Read the model definition and answer for the solid it produces. Units are mm, in the model's axes. Face numbers are marked on the shaded views. A direction names the side the tool comes from. Give positions to 0.01 mm unless a question says otherwise; leave off trailing zeros. Order: outer loops, then holes, each group sorted by start corner. A loop starts at its lowest first (then second) coordinate and runs counter-clockwise, first axis right, second up.
```python
from build123d import *

# Parameters (mm, degrees)
ESTRUSIONE_ESTRUSIONE1_DEPTH = 70
SCHIZZO2_W                   = 40
SCHIZZO2_H                   = 4.3
ESTRUSIONE_ESTRUSIONE2_DEPTH = 4.8


with BuildPart() as part:
    # Schizzo1 → Estrusione-Estrusione1 (new body)
    with BuildSketch(Plane(origin=(0, 0, 0), x_dir=(0, 0, -1), z_dir=(1, 0, 0))):
        Polygon((-61.1, 64.5), (-61.1, 19.5), (-49.6, 19.5), (-49.6, 11), (-29.6, 11), (-29.6, 0), (0, 0), (0, 24), (-4.3, 24), (-4.3, 59.5), (0, 59.5), (0, 73), (-4.3, 84), (-29.6, 84), (-29.6, 73), (-49.6, 73), (-49.6, 64.5), align=None)
    extrude(amount=ESTRUSIONE_ESTRUSIONE1_DEPTH)

    # Schizzo2 → Estrusione-Estrusione2 (add)
    with BuildSketch(Plane.XZ):
        with Locations((35, 2.15)):
            Rectangle(SCHIZZO2_W, SCHIZZO2_H)
    extrude(amount=ESTRUSIONE_ESTRUSIONE2_DEPTH)


solid = part.part
```
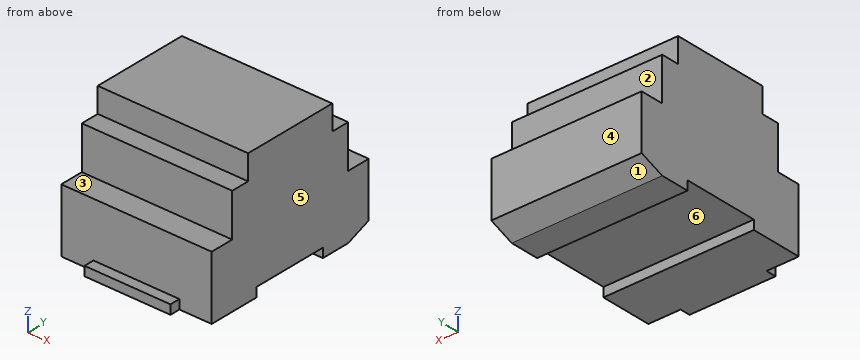
1) The part is cut by section C-C on z = 26. Determine the outline of the cut face in (x, y), and give its area (3 significant figures).
Final values:
outline: (0, 0) - (70, 0) - (70, 84) - (0, 84) - close
area: 5,880 mm2
2) The part is cut by section D-D on x = 30. Determine the outline of the cut face in (y, z), and give its area (3 significant figures).
Final values:
outline: (-4.8, 0) - (24, 0) - (24, 4.3) - (59.5, 4.3) - (59.5, 0) - (73, 0) - (84, 4.3) - (84, 29.6) - (73, 29.6) - (73, 49.6) - (64.5, 49.6) - (64.5, 61.1) - (19.5, 61.1) - (19.5, 49.6) - (11, 49.6) - (11, 29.6) - (0, 29.6) - (0, 4.3) - (-4.8, 4.3) - close
area: 4,090 mm2
3) Given pin 1 (9 mm diameter, centred on x = 42.5, z = 13, fed in from -Y); pin 2 (16 mm diameter, centred on x = 21, z = 40.5, fed in from -Y); pin 3 (3 mm diameter, centred on x = 21, y = 9, fed in from +Z); pin 4 (10 mm diameter, centred on y = 56.5, z = 20, fed in from -X), each flat-ended and moving along its own axis, determine where each tip first touches the part or whether it passes through.
Final values:
pin 1: stops at y = 0
pin 2: stops at y = 11
pin 3: stops at z = 29.6
pin 4: stops at x = 0
4) The part is cut by section B-B on y = 31.5. Determine the outline of the cut face in (x, z).
Final values:
outline: (0, 4.3) - (70, 4.3) - (70, 61.1) - (0, 61.1) - close
5) For a pull along Y with two mould halves and no side action, classify the marked faces 4, 5 and 6 as released by +Y, released by -Y, zero draft, split by the parting line, or undercut.
Final values:
face 4: released by +Y
face 5: zero draft
face 6: undercut
6) A tool of negligible diameter and unlimited length cuts with its end or side. For the marked faces 1, 2 and 3, from which of +Z, -Z, +X, -X, +Y, -Y can it reach the whole face along a straight path? Write none if from no direction.
Final values:
face 1: -Z, +X, -X, +Y
face 2: +Z, +X, -X, +Y
face 3: +Z, +X, -X, -Y
7) Consider L1, parallel to Y at x = 7, z = 22; L2, parallel to Z at x = 48, y = 59; L3, parallel to Z at x = 15, y = 4. Determine where each line is inside the solid, lowest interval first.
Final values:
L1: y = 0 to 84
L2: z = 4.3 to 61.1
L3: z = 0 to 29.6
8) The part is cut by section A-A on x = 13. Determine the outline of the cut face in (y, z), and give its area (3 significant figures).
Final values:
outline: (0, 0) - (24, 0) - (24, 4.3) - (59.5, 4.3) - (59.5, 0) - (73, 0) - (84, 4.3) - (84, 29.6) - (73, 29.6) - (73, 49.6) - (64.5, 49.6) - (64.5, 61.1) - (19.5, 61.1) - (19.5, 49.6) - (11, 49.6) - (11, 29.6) - (0, 29.6) - close
area: 4,070 mm2
